Can you work these out from the model? Positions are in its coordinate system, mm. Round coordinates to 2 decimals unless told otherwise and drop trailing zeros. Write each loop counter-clockwise with the first axis right and the second up, starting at its lowest first coordinate (ties: lowest second). Pieces come first, ordered by that corner, then holes.
Q1. If we section it at B-B (x = -30): Please give me the cut outline in (y, z), plus the area to 3 significant figures.
Q2. Please list where these lines run through material, in increasing order: line 1 along X through (y, z) = (0.45, -23.2); line 2 along X through (y, z) = (0.35, -21.9); line 3 along Z through (x, y) = (-27, 0.45).
Q3. If we section it at A-A (z = -23.4): Please give me the cut outline in (x, y).
Q4. If we section it at D-D (x = -26.5): Please give me the cut outline in (y, z).
Q5. If we section it at C-C (y = 0.15): Please give me the cut outline in (x, z).
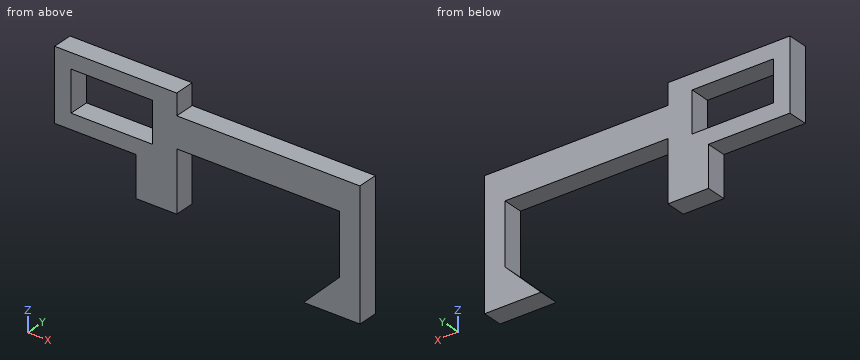
from build123d import *

# Parameters (mm, degrees)
BOSS_EXTRUDE1_DEPTH = 0.5


with BuildPart() as part:
    # Sketch1 → Boss-Extrude1 (new body)
    with BuildSketch(Plane(origin=(0, 0, 0), x_dir=(1, 0, 0), z_dir=(0, 1, 0))):
        Polygon((-23.973296771, 22.315949047), (-27.973296771, 22.315949047), (-27.973296771, 23.798880368), (-28.973178979, 23.798880368), (-28.973178979, 22.798880368), (-30.973296771, 22.798880368), (-30.973296771, 21.923880368), (-30.973296771, 21.048880368), (-27.973296771, 21.048880368), (-27.973296771, 21.565949047), (-23.473296771, 21.565949047), (-23.473296771, 24.699832523), (-24.857180247, 24.699832523), (-23.973296771, 23.815949047), align=None)
        Polygon((-30.569749298, 21.423880368), (-30.569749298, 21.923880368), (-30.569749298, 22.423880368), (-28.569749298, 22.423880368), (-28.569749298, 21.423880368), align=None, mode=Mode.SUBTRACT)
    extrude(amount=BOSS_EXTRUDE1_DEPTH)


solid = part.part
A:
1. outline: (0, -22.8) - (0.5, -22.8) - (0.5, -22.42) - (0, -22.42) - close; (0, -21.42) - (0.5, -21.42) - (0.5, -21.05) - (0, -21.05) - close
1. area: 0.375 mm2
2. line 1: x = -28.97 to -27.97, -23.97 to -23.47
2. line 2: x = -30.97 to -30.57, -28.57 to -23.47
2. line 3: z = -22.32 to -21.57
3. outline: (-28.97, 0) - (-27.97, 0) - (-27.97, 0.5) - (-28.97, 0.5) - close; (-23.97, 0) - (-23.47, 0) - (-23.47, 0.5) - (-23.97, 0.5) - close
4. outline: (0, -22.32) - (0.5, -22.32) - (0.5, -21.57) - (0, -21.57) - close
5. outline: (-30.97, -22.8) - (-28.97, -22.8) - (-28.97, -23.8) - (-27.97, -23.8) - (-27.97, -22.32) - (-23.97, -22.32) - (-23.97, -23.82) - (-24.86, -24.7) - (-23.47, -24.7) - (-23.47, -21.57) - (-27.97, -21.57) - (-27.97, -21.05) - (-30.97, -21.05) - close; hole (-30.57, -22.42) - (-28.57, -22.42) - (-28.57, -21.42) - (-30.57, -21.42) - close
